Autodesk Inventor part; units mm, degrees
ref_plane "YZ Plane" through (0, 0, 0) normal (1, 0, 0) x (0, 1, 0)
ref_plane "XZ Plane" through (0, 0, 0) normal (0, 1, 0) x (-1, 0, 0)
ref_plane "XY Plane" through (0, 0, 0) normal (0, 0, 1) x (1, 0, 0)
sketch "Sketch1" plane through (0, 0, 0) normal (0, 0, 1) x (1, 0, 0)
  line L0 (-42.1338, 2.3056) -> (122.9662, 2.3056)
  line L1 (122.9662, 2.3056) -> (122.9662, -4.0444)
  line L2 (122.9662, -4.0444) -> (-42.1338, -4.0444)
  line L3 (-42.1338, -4.0444) -> (-42.1338, 2.3056)
  line L4 (-42.1338, 2.3056) -> (-42.1338, -0.8694)
  line L5 (-42.1338, -0.8694) -> (122.9662, -0.8694)
  circle A0 centre (-42.1338, -0.8694) radius 3.175
  circle A1 centre (122.9662, -0.8694) radius 3.175
  point P0 (0, 0)
  dimension "d0" = 165.1
  dimension "d1" = 6.35
extrude "Extrusion1" add sketch "Sketch1" along normal blind 3.175
sketch "Sketch2" plane through (0, 0, 3.175) normal (0, 0, 1) x (1, 0, 0)
  arc A0 (122.9662, -4.0444) -> (122.9662, 2.3056) centre (122.9662, -0.8694) ccw
  arc A1 (-42.1338, 2.3056) -> (-42.1338, -4.0444) centre (-42.1338, -0.8694) ccw
  circle A2 centre (-42.1338, -0.8694) radius 3.175
  circle A3 centre (122.9662, -0.8694) radius 6.35
  circle A4 centre (-42.1338, -0.8694) radius 6.35
  circle A5 centre (122.9662, -0.8694) radius 3.175
  point P0 (0, 0)
  dimension "d4" = 12.7
  dimension "d5" = 12.7
extrude "Extrusion2" cut sketch "Sketch2" against normal blind 3.175 contours A5 A0 | A2 A1
sketch "Sketch3" plane through (0, 0, 3.175) normal (0, 0, 1) x (1, 0, 0)
  arc A0 (122.9662, 2.3056) -> (122.9662, -4.0444) centre (122.9662, -0.8694) ccw
  arc A1 (-42.1338, -4.0444) -> (-42.1338, 2.3056) centre (-42.1338, -0.8694) ccw
  circle A2 centre (-42.1338, -0.8694) radius 3.175
  circle A3 centre (-42.1338, -0.8694) radius 6.35
  circle A4 centre (122.9662, -0.8694) radius 3.175
  circle A5 centre (122.9662, -0.8694) radius 6.35
  point P0 (0, 0)
  dimension "d8" = 12.7
  dimension "d9" = 12.7
extrude "Extrusion3" add sketch "Sketch3" against normal blind 3.175
properties part number "bar2"
The model under review builds one solid part; all positions refer to its coordinate system, in mm. Round coordinates to 2 decimals unless told otherwise and drop trailing zeros. Loops run counter-clockwise (first coordinate to the right, second up) from the corner with the lowest first, then second, coordinate; pieces in that order, holes last. Notation, with made-up numbers: (88.25, -15.75) - (95.25, -15.75) arc R14 cw to (95.25, -6.75) - close; hole circle Ø7 at (3.5, -28.75). An arc over 180 degrees is marked (long way). Write each question's results on one line, items separated by ' | '. Start each with the question number.
Q1. Take a section at C-C on x = -25. Give the boundary of the cut face in (y, z) (3 decimals).
Q2. Wall thickness on line 1 along X through (y, z) = (-0.75, 1.8); line 2 along X through (y, z) = (-3.25, 1.95); line 3 along Y through (x, z) = (12, 1.2): over which ranges is each line inside the solid? List them lowest first. Write a range as [from, to].
Q3. Draft analysis for pull direction Y (two halves, no side actions). For faces 1 (the cylindrical face through (-39.034, -1.558, 1.61)), 2 (the flat face through (41, -4.044, 2)), 3 (the flat face through (39, 2.306, 2)), 4 (the flat face through (39, -1, 3.175)), state which applies: pulls with the +Y half, pulls with the -Y half, needs draft (parallel to the pull), parting line crosses it, or undercut.
Q4. Insertion check: P1, Ø1.6, axis at x = 61.5, z = 2, coming from the +Y side. The pin has a flat end and moves straight along its axis. Give the tip position at first contact, or say it passes through.
Q5. Take a section at B-B on z = 0.8. Give the boundary of the cut face in (x, y) (3 decimals).
Q6. Take a section at A-A on y = 3.75. Give the boundary of the cut face in (x, z) (3 decimals).
Data:
1) outline: (-4.044, 0) - (2.306, 0) - (2.306, 3.175) - (-4.044, 3.175) - close
2) line 1: x = [-48.48, -45.31], [-38.96, 119.79], [126.14, 129.32] | line 2: x = [-48.02, -44.23], [-40.03, 120.87], [125.07, 128.85] | line 3: y = [-4.04, 2.31]
3) face 1: undercut | face 2: pulls with the -Y half | face 3: pulls with the +Y half | face 4: needs draft
4) P1: stops at y = 2.31
5) outline: (-36.635, -4.044) - (117.467, -4.044) arc R6.35 ccw (long way) to (117.467, 2.306) - (-36.635, 2.306) arc R6.35 ccw (long way) to start; hole circle Ø6.35 at (-42.134, -0.869); hole circle Ø6.35 at (122.966, -0.869)
6) outline: (-46.491, 0) - (-37.777, 0) - (-37.777, 3.175) - (-46.491, 3.175) - close; (118.609, 0) - (127.323, 0) - (127.323, 3.175) - (118.609, 3.175) - close
